from build123d import *

# Parameters (mm, degrees)
F0_W     = 3
F0_H     = 10
F1_DEPTH = 5
F2_W     = 45
F2_H     = 10
F2_W_2   = 3
F3_DEPTH = 1


with BuildPart() as f1:
    # F0 (on Top) → F1 (new body)
    with BuildSketch(Plane.XY):
        with Locations((-26.961136, -5)):
            Rectangle(F0_W, F0_H)
        with Locations((-21.961136, -5)):
            Rectangle(F0_W, F0_H)
        with Locations((-14.961136, -5)):
            Rectangle(F0_W, F0_H)
        with Locations((-5.961136, -5)):
            Rectangle(F0_W, F0_H)
        with Locations((5.038864, -5)):
            Rectangle(F0_W, F0_H)
        with Locations((18.038864, -5)):
            Rectangle(F0_W, F0_H)
    extrude(amount=F1_DEPTH)

    # F2 (on face) → F3 (join)
    with BuildSketch(Plane(origin=(0, 0, 0), x_dir=(1, 0, 0), z_dir=(0, 0, -1))):
        with Locations((-2.961136, 5)):
            Rectangle(F2_W, F2_H)
        with Locations((-26.961136, 5)):
            Rectangle(F2_W_2, F2_H)
    extrude(amount=F3_DEPTH)


solid = f1.part
The model under review builds one solid part; all positions refer to its coordinate system, in mm. A direction names the side the tool comes from. Round coordinates to 2 decimals unless told otherwise and drop trailing zeros. Order: outer loops, then holes, each group sorted by start corner. A loop starts at its lowest first (then second) coordinate and runs counter-clockwise, first axis right, second up. Notation, with made-up numbers: (-3.5, 13) -> (21.5, 13) arc R24 cw to (21.5, 32) -> close; hole circle Ø6 at (-18.75, 18.5). An arc over 180 degrees is marked (long way). Write item = value, one per line. Start each with the question number.
Item 1: Mouldability with a two-part tool opening along X and no side actions: class faces 1 (the face through (-28.461, -5, 2)), 2 (the face through (-16.461, -5, 2)), 3 (the face through (19.539, -5, 2)), 4 (the face through (-25.461, -5, 2)) as released by +X, released by -X, zero draft, split by the parting line, or undercut.
Item 2: Consider section A-A on z = 4. Write out the cut boundary in (x, y), plus the area to 3 significant figures.
Item 3: For line 1 along X through (y, z) = (-4.25, 0.25); line 2 along Z through (x, y) = (-2, -0.5), list the stretches that pass through material, from the lowest coordinate up.
Item 4: Clearance check with a flat-ended pin moving along its axis: pin 1 Ø3 at (x, y) = (12.5, -4) entering from +Z. State where the tip first meets the part, or that it passes through.
Item 5: Consider section C-C on x = 12.5. Write out the cut boundary in (y, z).
Item 6: For faces 5 (the face through (5, -5, 5)), 6 (the face through (16.539, -5, 2)), list the 3-axis set-ups (+Z, -Z, +X, -X, +Y, -Y) from which the entire face can be reached by the end or side of a thin tool; tool diameter is ignored.
Item 7: Consider section B-B on y = -8.75. Write out the cut boundary in (x, z).
Conclusion:
q1.face_1 = released by -X
q1.face_2 = undercut
q1.face_3 = released by +X
q1.face_4 = undercut
q2.outline = (-28.46, -10) -> (-25.46, -10) -> (-25.46, 0) -> (-28.46, 0) -> close; (-23.46, -10) -> (-20.46, -10) -> (-20.46, 0) -> (-23.46, 0) -> close; (-16.46, -10) -> (-13.46, -10) -> (-13.46, 0) -> (-16.46, 0) -> close; (-7.46, -10) -> (-4.46, -10) -> (-4.46, 0) -> (-7.46, 0) -> close; (3.54, -10) -> (6.54, -10) -> (6.54, 0) -> (3.54, 0) -> close; (16.54, -10) -> (19.54, -10) -> (19.54, 0) -> (16.54, 0) -> close
q2.area = 180 mm2
q3.line_1 = -28.46 to -25.46, -23.46 to -20.46, -16.46 to -13.46, -7.46 to -4.46, 3.54 to 6.54, 16.54 to 19.54
q3.line_2 = -1 to 0
q4.pin_1 = 0
q5.outline = (-10, -1) -> (0, -1) -> (0, 0) -> (-10, 0) -> close
q6.face_5 = +Z, +X, -X, +Y, -Y
q6.face_6 = +Z, +Y, -Y
q7.outline = (-28.46, -1) -> (19.54, -1) -> (19.54, 5) -> (16.54, 5) -> (16.54, 0) -> (6.54, 0) -> (6.54, 5) -> (3.54, 5) -> (3.54, 0) -> (-4.46, 0) -> (-4.46, 5) -> (-7.46, 5) -> (-7.46, 0) -> (-13.46, 0) -> (-13.46, 5) -> (-16.46, 5) -> (-16.46, 0) -> (-20.46, 0) -> (-20.46, 5) -> (-23.46, 5) -> (-23.46, 0) -> (-25.46, 0) -> (-25.46, 5) -> (-28.46, 5) -> close
